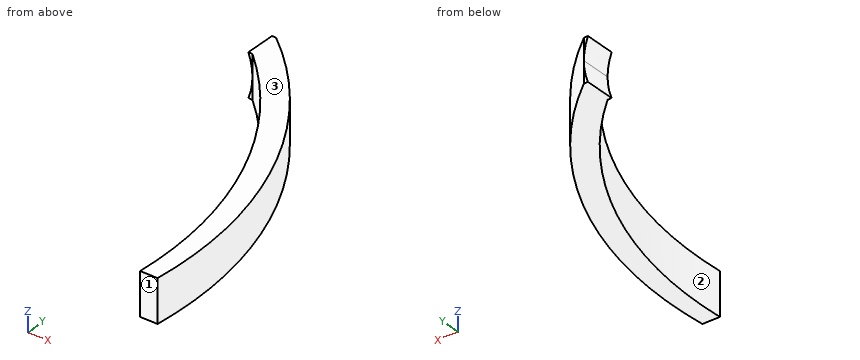
from build123d import *

# Parameters (mm, degrees)
BOSS_EXTRUDE1_DEPTH = 10
BOSS_EXTRUDE2_DEPTH = 7


with BuildPart() as part:
    # Sketch1 → Boss-Extrude1 (new body)
    with BuildSketch(Plane.XY):
        with BuildLine():
            Line((-18.757439303, 33.418117649), (-18.925359206, 26.418117649))
            ThreePointArc((-18.925359206, 26.418117649), (3.268987797, -5.966966431), (8.965935836, -44.811882351))
            Line((8.965935836, -44.811882351), (12.965935836, -44.811882351))
            ThreePointArc((12.965935836, -44.811882351), (7.097147968, -1.644619716), (-18.757439303, 33.418117649))
        make_face()
    extrude(amount=BOSS_EXTRUDE1_DEPTH)

    # Sketch2 → Boss-Extrude2 (add)
    with BuildSketch(Plane(origin=(0.790403617, 32.949193093, 0), x_dir=(0, 0, -1), z_dir=(0.02398165846895122, 0.9997123986712771, 0))):
        with BuildLine():
            Line((-10, 20.513530318), (-10, 19.553466522))
            Line((-10, 19.553466522), (-5, 19.553466522))
            ThreePointArc((-5, 19.553466522), (-7.545668993, 19.795654886), (-10, 20.513530318))
        make_face()
        with BuildLine():
            ThreePointArc((0, 20.513530318), (-2.454331007, 19.795654886), (-5, 19.553466522))
            Line((-5, 19.553466522), (0, 19.553466522))
            Line((0, 19.553466522), (0, 20.513530318))
        make_face()
    extrude(amount=-BOSS_EXTRUDE2_DEPTH)


solid = part.part
For this review, take the finished solid that the model builds, in its own axes (mm). Face numbers are marked on the shaded views. Round coordinates to 2 decimals unless told otherwise and drop trailing zeros. Order: outer loops, then holes, each group sorted by start corner. A loop starts at its lowest first (then second) coordinate and runs counter-clockwise, first axis right, second up. Notation, with made-up numbers: M 64.5,-25.75 L 87.5,-25.75 A26 ccw 87.5,9.25 Z; hole C 39.5,56 d8. An arc over 180 degrees is marked long. Use a Markdown table: item, result. Add a question column.
Item 1: To check wall thickness, follow line 1 along X through (y, z) = (-24, 4); line 2 along Y through (x, z) = (-2, 6.5); line 3 along Y through (x, z) = (-17, 6.25). State the ranges of each line that lie inside material, in increasing order.
Item 2: Mouldability with a two-part tool opening along Y and no side actions: class the marked faces 1, 2 and 3 as released by +Y, released by -Y, zero draft, split by the parting line, or undercut.
Item 3: Add section C-C, the plane x = 4.5. Give the boundary of the cut face in (y, z).
Item 4: Add section B-B, the plane y = -38.5. Give the boundary of the cut face in (x, z), then the cut area to 3 significant figures.
Item 5: Insertion check: pin 1 (5 mm diameter, centred on x = 6, y = 11.5, fed in from +Z); pin 2 (1 mm diameter, centred on x = -9.5, z = 1.5, fed in from +Y); pin 3 (1.5 mm diameter, centred on x = 2, z = 3.5, fed in from +Y); pin 4 (1.5 mm diameter, centred on y = 18.5, z = 8.5, fed in from +X). Each pin has a flat end and moves straight along its axis. Give the tip position at first contact, or say it passes through.
Geometry results:
| question | item | result |
|---|---|---|
| 1 | line 1 | x = 8.17 to 12.89 |
| 1 | line 2 | y = 5.12 to 15.23 |
| 1 | line 3 | y = 24.6 to 31.94 |
| 2 | face 1 | released by -Y |
| 2 | face 2 | undercut |
| 2 | face 3 | zero draft |
| 3 | outline | M -9.31,0 L 4.15,0 L 4.15,10 L -9.31,10 Z |
| 4 | outline | M 9.25,0 L 13.47,0 L 13.47,10 L 9.25,10 Z |
| 4 | area | 42.1 mm² |
| 5 | pin 1 | passes through |
| 5 | pin 2 | stops at y = 25.2 |
| 5 | pin 3 | stops at y = 10.15 |
| 5 | pin 4 | stops at x = -3.8 |
